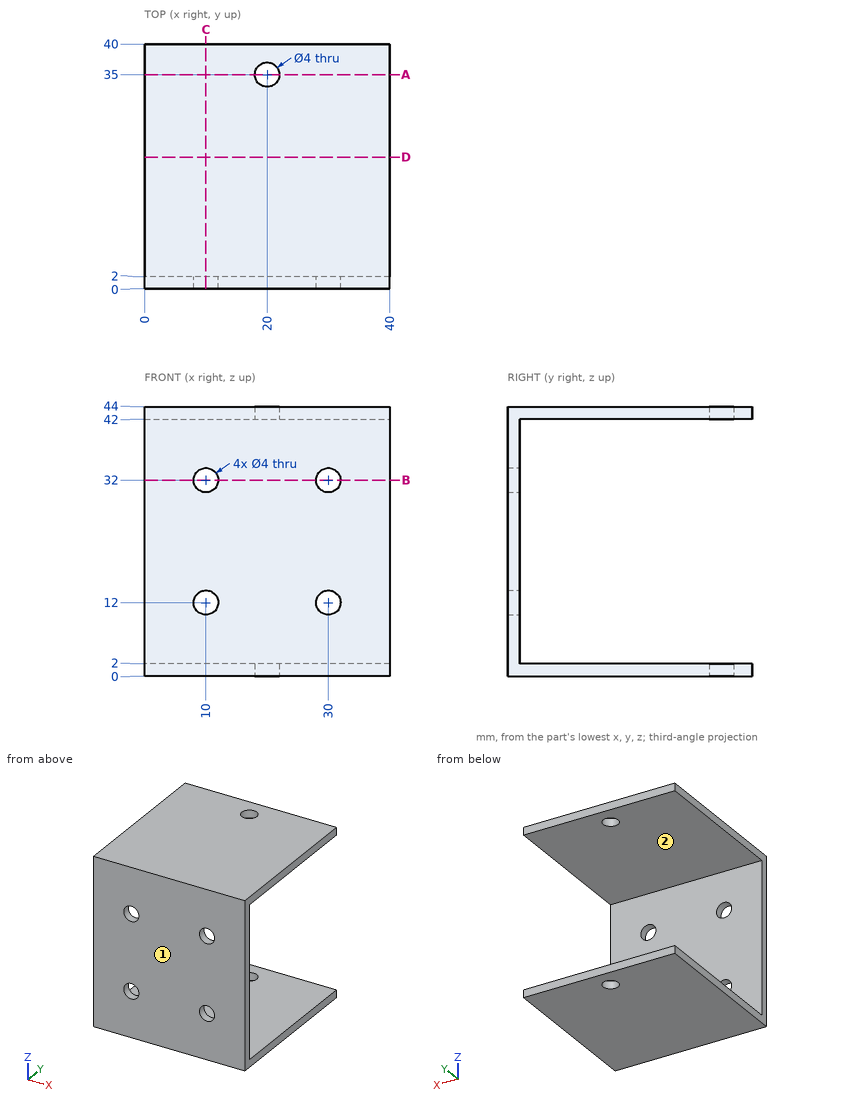
Geometry check sheet. Reference: drawing and pictorial views, mm from the part's lowest x, y, z. A direction names the side the tool comes from. Coordinates: 2 decimals unless noted, no trailing zeros. Loops run counter-clockwise (first coordinate to the right, second up) from the corner with the lowest first, then second, coordinate; pieces in that order, holes last. Notation, with made-up numbers: (-32, 31.25) -> (-22, 31.25) arc R20 cw to (-22, 59.25) -> close; hole circle Ø9 at (27.25, -11). An arc over 180 degrees is marked (long way). Write item = value, one per line. Start each with the question number.
1. Section check B-B on z = 32. Record the cut outline in (x, y), then the cut area to 3 significant figures.
2. Depth check by flat-ended pin: P1, Ø5, axis at x = 30, z = 32, coming from the +Y side. Enter the tip coordinate at first touch or a pass-through.
3. Section check C-C on x = 10. Record the cut outline in (y, z).
4. Section check D-D on y = 21.5. Record the cut outline in (x, z).
5. Section check A-A on y = 35. Record the cut outline in (x, z), then the cut area to 3 significant figures.
6. Tool access check on the marked faces 1 and 2. Record the directions out of +Z, -Z, +X, -X, +Y, -Y that give a thin tool (end or side, any length) a straight path to the whole face; none if there is none.
7. Material ranges on line 1 (Z direction, x = 10, y = 1); line 2 (X direction, y = 0.55, z = 12); line 3 (Z direction, x = 7, y = 31), recorded low to high.
Responses:
q1.outline = (0, 0) -> (8, 0) -> (8, 2) -> (0, 2) -> close; (12, 0) -> (28, 0) -> (28, 2) -> (12, 2) -> close; (32, 0) -> (40, 0) -> (40, 2) -> (32, 2) -> close
q1.area = 64.0 mm2
q2.P1 = 2
q3.outline = (0, 0) -> (40, 0) -> (40, 2) -> (2, 2) -> (2, 10) -> (0, 10) -> close; (0, 14) -> (2, 14) -> (2, 30) -> (0, 30) -> close; (0, 34) -> (2, 34) -> (2, 42) -> (40, 42) -> (40, 44) -> (0, 44) -> close
q4.outline = (0, 0) -> (40, 0) -> (40, 2) -> (0, 2) -> close; (0, 42) -> (40, 42) -> (40, 44) -> (0, 44) -> close
q5.outline = (0, 0) -> (18, 0) -> (18, 2) -> (0, 2) -> close; (0, 42) -> (18, 42) -> (18, 44) -> (0, 44) -> close; (22, 0) -> (40, 0) -> (40, 2) -> (22, 2) -> close; (22, 42) -> (40, 42) -> (40, 44) -> (22, 44) -> close
q5.area = 144 mm2
q6.face_1 = +Z, -Z, +X, -X, -Y
q6.face_2 = +X, -X, +Y
q7.line_1 = 0 to 10, 14 to 30, 34 to 44
q7.line_2 = 0 to 8, 12 to 28, 32 to 40
q7.line_3 = 0 to 2, 42 to 44
